Design review of the part built by this model. Coordinates are the model's own, in mm. Face numbers are marked on the shaded views. A direction names the side the tool comes from. Round coordinates to 2 decimals unless told otherwise and drop trailing zeros. Order: outer loops, then holes, each group sorted by start corner. A loop starts at its lowest first (then second) coordinate and runs counter-clockwise, first axis right, second up. Notation, with made-up numbers: (23.25, 7.25) - (62.25, 7.25) arc R20 cw to (62.25, 42.25) - close; hole circle Ø1 at (35, 67.25). An arc over 180 degrees is marked (long way). Answer as a JSON object with one key per item and string values. Group by question number.
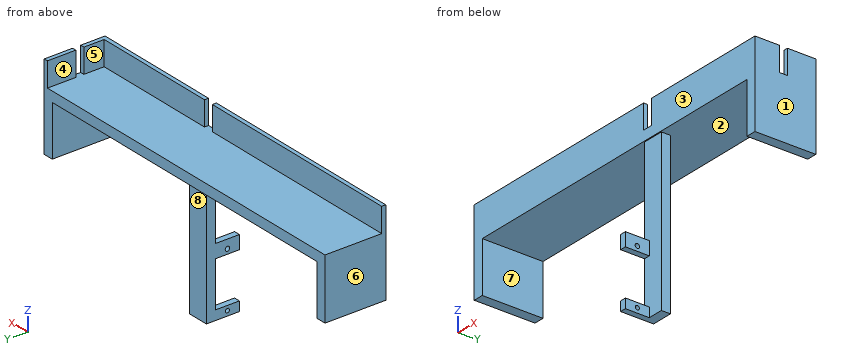
Autodesk Fusion 360 part; units mm, degrees
sketch "Sketch2" plane through (0, 0, 0) normal (0, 1, 0) x (1, 0, 0)
  line L0 (0, -62.2369) -> (87.5, -62.2369)
  line L1 (87.5, -62.2369) -> (87.5, -32.2369)
  line L2 (87.5, -32.2369) -> (82.5, -32.2369)
  line L3 (0, -57.2369) -> (0, -62.2369)
  line L4 (82.5, -32.2369) -> (82.5, -57.2369)
  line L5 (82.5, -57.2369) -> (0, -57.2369)
  line L6 (0, 0) -> (0, -57.2369) construction
  line L7 (-87.5, -32.2369) -> (-82.5, -32.2369)
  line L8 (-82.5, -32.2369) -> (-82.5, -57.2369)
  line L9 (-82.5, -57.2369) -> (0, -57.2369)
  line L10 (0, -57.2369) -> (0, -62.2369)
  line L11 (0, -62.2369) -> (-87.5, -62.2369)
  line L12 (-87.5, -62.2369) -> (-87.5, -32.2369)
  line L13 (0, 0) -> (30, 0) construction
  line L14 (0, 0) -> (0, -10.6) construction
  line L15 (18, 21.3) -> (28.4945, 21.3)
  line L16 (28.4945, 21.3) -> (28.4945, -57.2369)
  line L17 (28.4945, -57.2369) -> (18, -57.2369)
  line L18 (18, -57.2369) -> (18, 21.3)
  line L19 (21, -10.6) -> (18, -10.6)
  line L20 (18, -10.6) -> (18, -5.9)
  line L21 (18, -5.9) -> (21, -5.9)
  line L22 (21, -5.9) -> (21, -10.6)
  line L23 (0, 0) -> (0, 21.3) construction
  line L24 (18, 21.3) -> (21, 21.3)
  line L25 (21, 21.3) -> (21, 16.6)
  line L26 (21, 16.6) -> (18, 16.6)
  line L27 (18, 16.6) -> (18, 21.3)
  dimension "d1" = 5
  dimension "d2" = 82.5
  dimension "d3" = 5
  dimension "d4" = 25
  dimension "d10" = 10.6
  dimension "d14" = 4.7
  dimension "d15" = 3
  dimension "d16" = 21.3
  dimension "d17" = 3
  dimension "d18" = 4.7
  dimension "d19" = 22.5
extrude "Extrude1" add sketch "Sketch2" along normal blind 25 and the other way blind 5 contours L0 L1 L2 L3 L4 L5 L10 L17 | L3 L7 L8 L9 L10 L11 L12
extrude "Extrude2" add sketch "Sketch2" against normal blind 4.5 contours L5 L15 L16 L17 L18 L19 L21 L22 L25 L26 | L18 L19 L20 L21 L22 | L15 L18 L24 L25 L26 L27
extrude "Extrude3" add sketch "Sketch2" against normal blind 11.8 from surface at -4.5 contours L18 L19 L20 L21 L22 | L15 L18 L24 L25 L26 L27
sketch "Sketch3" plane through (21, 0, 0) normal (1, 0, 0) x (0, 1, 0)
  line L0 (-4.5, 5.9) -> (-4.5, 10.6)
  line L1 (-4.5, 10.6) -> (-16.3, 10.6)
  line L2 (-16.3, 10.6) -> (-16.3, 5.9)
  line L3 (-16.3, 5.9) -> (-4.5, 5.9)
  line L4 (-16.3, 10.6) -> (-10.4, 10.6) construction
  line L5 (-10.4, 10.6) -> (-10.4, 8.3) construction
  line L6 (-10.4, 8.3) -> (-16.3, 8.3) construction
  line L7 (-16.3, 8.3) -> (-16.3, 10.6) construction
  circle A0 centre (-10.4, 8.3) radius 1.1
  dimension "d23" = 5.9
  dimension "d24" = 2.3
  dimension "d25" = 2.2
sketch "Sketch4" plane through (21, 0, 0) normal (1, 0, 0) x (0, 1, 0)
  line L0 (-4.5, -21.3) -> (-4.5, -16.6)
  line L1 (-4.5, -16.6) -> (-16.3, -16.6)
  line L2 (-16.3, -16.6) -> (-16.3, -21.3)
  line L3 (-16.3, -21.3) -> (-4.5, -21.3)
  line L4 (-16.3, -16.6) -> (-10.4, -16.6) construction
  line L5 (-10.4, -16.6) -> (-10.4, -18.9) construction
  line L6 (-10.4, -18.9) -> (-16.3, -18.9) construction
  line L7 (-16.3, -18.9) -> (-16.3, -16.6) construction
  circle A0 centre (-10.4, -18.9) radius 1
  dimension "d26" = 5.9
  dimension "d27" = 2.3
  dimension "d28" = 2
extrude "Extrude4" cut sketch "Sketch4" against normal blind 6 contours A0
extrude "Extrude5" cut sketch "Sketch3" against normal blind 5.5 contours A0
extrude "Extrude6" add 1 faces at (20, -12.3667, 10.6) along direction (0, 0, 1) blind 2
sketch "Sketch5" plane through (0, 0, 62.2369) normal (0, 0, 1) x (-1, 0, 0)
  line L0 (-87.5, 5) -> (-87.5, -25)
  line L1 (-87.5, -25) -> (87.5, -25)
  line L2 (87.5, -25) -> (87.5, 5)
  line L3 (87.5, 5) -> (-87.5, 5)
  line L4 (87.5, 5) -> (-87.5, 5)
  line L5 (-87.5, 5) -> (-87.5, 3)
  line L6 (-87.5, 3) -> (87.5, 3)
  line L7 (87.5, 3) -> (87.5, 5)
  line L8 (-18.0867, 5) -> (-18.0867, 3)
  line L9 (-23.0002, 5) -> (-23.0002, 3)
  line L10 (-87.5, 3) -> (-85.5, 3)
  line L11 (-85.5, 3) -> (-85.5, -25)
  line L12 (-85.5, -25) -> (-87.5, -25)
  line L13 (-87.5, -25) -> (-87.5, 3)
  line L14 (-85.5, -11) -> (-87.5, -11)
  line L15 (-87.5, -11) -> (-87.5, -9)
  line L16 (-87.5, -9) -> (-85.5, -9)
  line L17 (-85.5, -9) -> (-85.5, -11)
  dimension "d35" = 2
  dimension "d38" = 2
extrude "Extrude7" add sketch "Sketch5" along normal blind 12 contours L0 L3 L4 L5 L6 L9 L10 | L2 L3 L4 L6 L7 L8
extrude "Extrude8" add sketch "Sketch5" along normal blind 12 contours L0 L6 L10 L11 L13 L16 | L0 L1 L11 L12 L13 L14
extrude "Extrude9" cut 1 faces at (86.8333, 9, 70.2369) along direction (0, -1, 0) blind 2
equation "d10 = 5.9 mm + 4.7 mm"
1. Tool access review of the marked faces 5, 6, 7 and 8: name each direction out of +Z, -Z, +X, -X, +Y, -Y from which nothing blocks a thin tool from reaching the whole face with its end or side.
2. Mouldability with a two-part tool opening along X and no side actions: class the marked faces 1, 2, 3 and 4 as pulls with the +X half, pulls with the -X half, needs draft (parallel to the pull), parting line crosses it, or undercut.
3. Clearance check with flat-ended pins moving along their axes: P1, Ø5, axis at y = -2, z = -3, coming from the +X side; P2, Ø1.6, axis at x = 87, z = 70, coming from the -Y side; P3, Ø2.5, axis at x = 84, y = 9.5, coming from the -Z side. State where each tip first meets the part, or that it passes through.
4. To check wall thickness, follow line 1 (X direction, y = 9, z = 32.5); line 2 (Z direction, x = 19.25, y = -10.4); line 3 (Z direction, x = -43.5, y = 12.5). State the ranges of each line that lie inside material, in increasing order. Write a range as from..to.
5. Take a section at B-B, the plane x = 56. Give the boundary of the cut face in (y, z).
6. Take a section at A-A, the plane y = 5. Give the boundary of the cut face in (x, z).
Response values:
{
 "1": {"face 5": "+Z, -X, +Y", "face 6": "+Z, -Z, -X, +Y, -Y", "face 7": "-Z, +Y, -Y", "face 8": "-Z, +Y"},
 "2": {"face 1": "pulls with the +X half", "face 2": "undercut", "face 3": "needs draft", "face 4": "pulls with the -X half"},
 "3": {"P1": "x = 28.49", "P2": "y = -5", "P3": "z = 32.24"},
 "4": {"line 1": "-87.5..-82.5, 82.5..87.5", "line 2": "-21.3..-19.9, -17.9..-16.6, 5.9..7.2, 9.4..12.6", "line 3": "57.24..62.24"},
 "5": {"outline": "(-5, 57.24) - (25, 57.24) - (25, 62.24) - (-3, 62.24) - (-3, 74.24) - (-5, 74.24) - close"},
 "6": {"outline": "(-87.5, 32.24) - (-82.5, 32.24) - (-82.5, 57.24) - (82.5, 57.24) - (82.5, 32.24) - (87.5, 32.24) - (87.5, 74.24) - (85.5, 74.24) - (85.5, 62.24) - (-87.5, 62.24) - close"}
}
